Check sheet for the modelled part. Datum: model origin and axes. Units: mm. Face numbers are marked on the shaded views. A direction names the side the tool comes from. Give positions to 0.01 mm unless a question says otherwise; leave off trailing zeros. Order: outer loops, then holes, each group sorted by start corner. A loop starts at its lowest first (then second) coordinate and runs counter-clockwise, first axis right, second up. Notation, with made-up numbers: M 43,35.25 L 101,35.25 A21 ccw 101,61.25 Z; hole C -32,39 d1. An arc over 180 degrees is marked long. Return JSON: item names as keys, results as strings. Group by question number.
from build123d import *

# Parameters (mm, degrees)
SKETCH1_R           = 8
BOSS_EXTRUDE1_DEPTH = 10.5
SKETCH2_R           = 3.85
BOSS_EXTRUDE2_DEPTH = 60
BOSS_EXTRUDE3_START = -9.6
BOSS_EXTRUDE3_DEPTH = 10
CUT_EXTRUDE1_START  = -9.6
SKETCH6_R           = 3.85
CUT_EXTRUDE1_DEPTH  = 9.6
BOSS_EXTRUDE4_DEPTH = 10
SKETCH8_R           = 4.5
BOSS_EXTRUDE5_DEPTH = 0.5
SKETCH9_R           = 3.85
BOSS_EXTRUDE6_DEPTH = 50.4
BOSS_EXTRUDE7_DEPTH = 43.5
SKETCH12_R          = 1.75
CUT_EXTRUDE2_DEPTH  = 10


with BuildPart() as part:
    # Sketch1 → Boss-Extrude1 (new body)
    with BuildSketch(Plane.XY):
        Circle(SKETCH1_R)
    extrude(amount=-BOSS_EXTRUDE1_DEPTH)

    # Sketch2 → Boss-Extrude2 (add)
    with BuildSketch(Plane(origin=(0, 0, -10.5), x_dir=(-1, 0, 0), z_dir=(0, 0, -1))):
        Circle(SKETCH2_R)
    extrude(amount=BOSS_EXTRUDE2_DEPTH)

    # Sketch3 → Boss-Extrude3 (add)
    with BuildSketch(Plane(origin=(0, 0, -70.5), x_dir=(-1, 0, 0), z_dir=(0, 0, -1)).offset(BOSS_EXTRUDE3_START)):
        Polygon((-6.07919536, 0.208287708), (-1.121971054, 0.860918669), (-1.774602015, 5.818142976), (0.208287708, 6.07919536), (0.860918669, 1.121971054), (5.818142976, 1.774602015), (6.07919536, -0.208287708), (1.121971054, -0.860918669), (1.774602015, -5.818142976), (-0.208287708, -6.07919536), (-0.860918669, -1.121971054), (-5.818142976, -1.774602015), align=None)
    extrude(amount=-BOSS_EXTRUDE3_DEPTH)

    # Sketch6 → Cut-Extrude1 (cut)
    with BuildSketch(Plane(origin=(0, 0, -70.5), x_dir=(-1, 0, 0), z_dir=(0, 0, -1)).offset(CUT_EXTRUDE1_START)):
        with Locations(Location((0, 0, 0), (0, 0, 172.44534936))):
            Circle(SKETCH6_R)
    extrude(amount=CUT_EXTRUDE1_DEPTH, mode=Mode.SUBTRACT)

    # Sketch7 → Boss-Extrude4 (add)
    with BuildSketch(Plane.XY):
        with BuildLine():
            Line((1.96204938, 72.362976461), (-7.07246692, 3.739012125))
            Line((-7.07246692, 3.739012125), (7.799206001, 1.781119242))
            Line((7.799206001, 1.781119242), (16.8337223, 70.405083577))
            ThreePointArc((16.8337223, 70.405083577), (10.376832281, 78.819866479), (1.96204938, 72.362976461))
        make_face()
    extrude(amount=-BOSS_EXTRUDE4_DEPTH)

    # Sketch8 → Boss-Extrude5 (add)
    with BuildSketch(Plane(origin=(0, 0, -10), x_dir=(-1, 0, 0), z_dir=(0, 0, -1))):
        with Locations(Location((-9.39788584, 71.384030019, 0), (0, 0, 180))):
            Circle(SKETCH8_R)
    extrude(amount=BOSS_EXTRUDE5_DEPTH)

    # Sketch9 → Boss-Extrude6 (add)
    with BuildSketch(Plane(origin=(0, 0, -10.5), x_dir=(-1, 0, 0), z_dir=(0, 0, -1))):
        with Locations(Location((-9.39788584, 71.384030019, 0), (0, 0, 180))):
            Circle(SKETCH9_R)
    extrude(amount=BOSS_EXTRUDE6_DEPTH)

    # Sketch11 → Boss-Extrude7 (add)
    with BuildSketch(Plane(origin=(0, 0, -10), x_dir=(-1, 0, 0), z_dir=(0, 0, -1))):
        Polygon((-2.951315217, 51.908863587), (-10.584845783, 50.903890222), (-9.318741718, 41.286875067), (-1.685211153, 42.291848431), align=None)
    extrude(amount=BOSS_EXTRUDE7_DEPTH)

    # Sketch12 → Cut-Extrude2 (cut)
    with BuildSketch(Plane(origin=(0, 0, -53.5), x_dir=(-1, 0, 0), z_dir=(0, 0, -1))):
        with Locations(Location((-6.135028468, 46.597869327, 0), (0, 0, 90))):
            Circle(SKETCH12_R)
    extrude(amount=-CUT_EXTRUDE2_DEPTH, mode=Mode.SUBTRACT)


solid = part.part
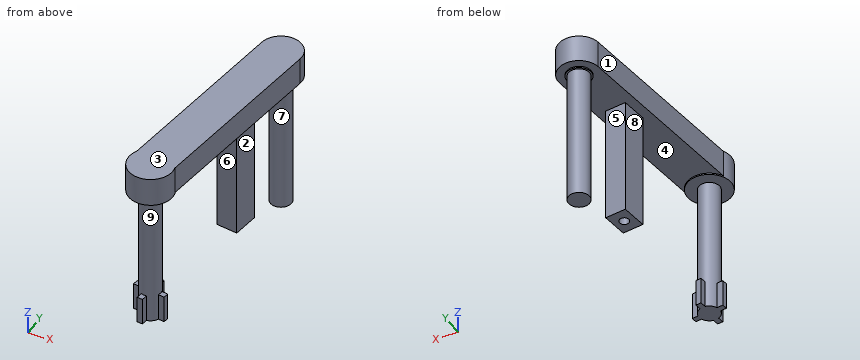
1) Sectioned sample at C-C on x = 15. Record the boundary of the cut face in (y, z), then the cut area to 3 significant figures.
2) Sectioned sample at A-A on z = -6. Record the boundary of the cut face in (x, y), then the cut area to 3 significant figures.
3) Tool access check on the marked faces 5, 6, 7, 8 and 9. Record the directions out of +Z, -Z, +X, -X, +Y, -Y that give a thin tool (end or side, any length) a straight path to the whole face; none if there is none.
4) Sectioned sample at B-B on z = -42.5. Record the boundary of the cut face in (x, y), then the cut area to 3 significant figures.
5) Depth check by flat-ended pin: P1, Ø3, axis at x = 6, y = 46.5, coming from the -Z side; P2, Ø6, axis at x = 4.5, z = -50, coming from the -Y side; P3, Ø7, axis at x = 5, y = 45.5, coming from the -Z side. Enter the tip coordinate at first touch or a pass-through.
6) Material ranges on line 1 along Y through (x, z) = (6, -50); line 2 along Z through (x, y) = (6.5, 64.5); line 3 along Z through (x, y) = (-2.75, 4), recorded low to high.
7) Release check for a two-part mould opening along Y. For the marked faces 1, 2, 3 and 4 record: released by +Y, released by -Y, zero draft, split by the parting line, or undercut.
Reply:
{
 "1": {"outline": "M 56.48,-10 L 76.37,-10 L 76.37,0 L 56.48,0 Z", "area": "199 mm^2"},
 "2": {"outline": "M -7.07,3.74 A8 ccw long 7.8,1.78 L 16.83,70.41 A7.5 ccw 1.96,72.36 Z", "area": "1,270 mm^2"},
 "3": {"face 5": "-Z, +X", "face 6": "-Z, -X", "face 7": "-Z", "face 8": "-Z, -X, +Y", "face 9": "none"},
 "4": {"outline": "C 0,0 d7.7; M 1.69,42.29 L 9.32,41.29 L 10.58,50.9 L 2.95,51.91 Z; C 9.4,71.38 d7.7", "area": "168 mm^2"},
 "5": {"P1": "z = -43.5", "P2": "y = -3.55", "P3": "z = -53.5"},
 "6": {"line 1": "41.72 to 44.85, 48.34 to 51.51, 69.57 to 73.19", "line 2": "-10 to 0", "line 3": "-10.5 to 0"},
 "7": {"face 1": "released by +Y", "face 2": "released by -Y", "face 3": "zero draft", "face 4": "undercut"}
}
